Input: dimensioned drawing with shaded views. Units: mm. Origin: part minimum x, y, z. A direction names the side the tool comes from. Coordinates: 2 decimals unless noted, no trailing zeros. Order: outer loops, then holes, each group sorted by start corner. A loop starts at its lowest first (then second) coordinate and runs counter-clockwise, first axis right, second up. Notation, with made-up numbers: (-7, 73.25) - (36, 73.25) arc R33 cw to (36, 104.25) - close; hole circle Ø2 at (4, 58.25). An arc over 180 degrees is marked (long way). Answer as CSV lines item,"result". Start each with the question number.
Item 1: Draft query along X for the marked faces 4, 5 and 6. Return one class per face: +X half, -X half, draft (parallel to the pull), parting line (faces both ways), or undercut.
Item 2: Material intervals for line 1 along Z through (x, y) = (45, 38); line 2 along X through (y, z) = (35, 41.5); line 3 along Z through (x, y) = (40.5, 67), sorted ascending.
Item 3: First-contact query: pin 1 (5 mm diameter, centred on x = 32.5, z = 25, fed in from +Y); pin 2 (3 mm diameter, centred on x = 32.5, z = 17.5, fed in from +Y); pin 3 (1 mm diameter, centred on y = 44.5, z = 10.5, fed in from -X); pin 4 (4 mm diameter, centred on x = 36.5, y = 51, fed in from -Z). Flat tips, straight axial feed; report the tip coordinate or a pass-through.
Item 4: Access query for the marked faces 1, 2 and 3. Directions: +Z, -Z, +X, -X, +Y, -Y. A direction counts if a zero-diameter tool reaches every point of the face in a straight line with its end or side. Return the directions, or none.
Item 5: Section C-C (x = 38.1). Output: boundary loops of the cut face in (y, z).
Item 6: Section B-B (y = 47.5). Output: boundary loops of the cut face in (x, z).
Item 7: Section A-A (z = 36). Output: boundary loops of the cut face in (x, y).
Item 8: Section D-D (z = 8). Output: boundary loops of the cut face in (x, y), and give its area (3 significant figures).
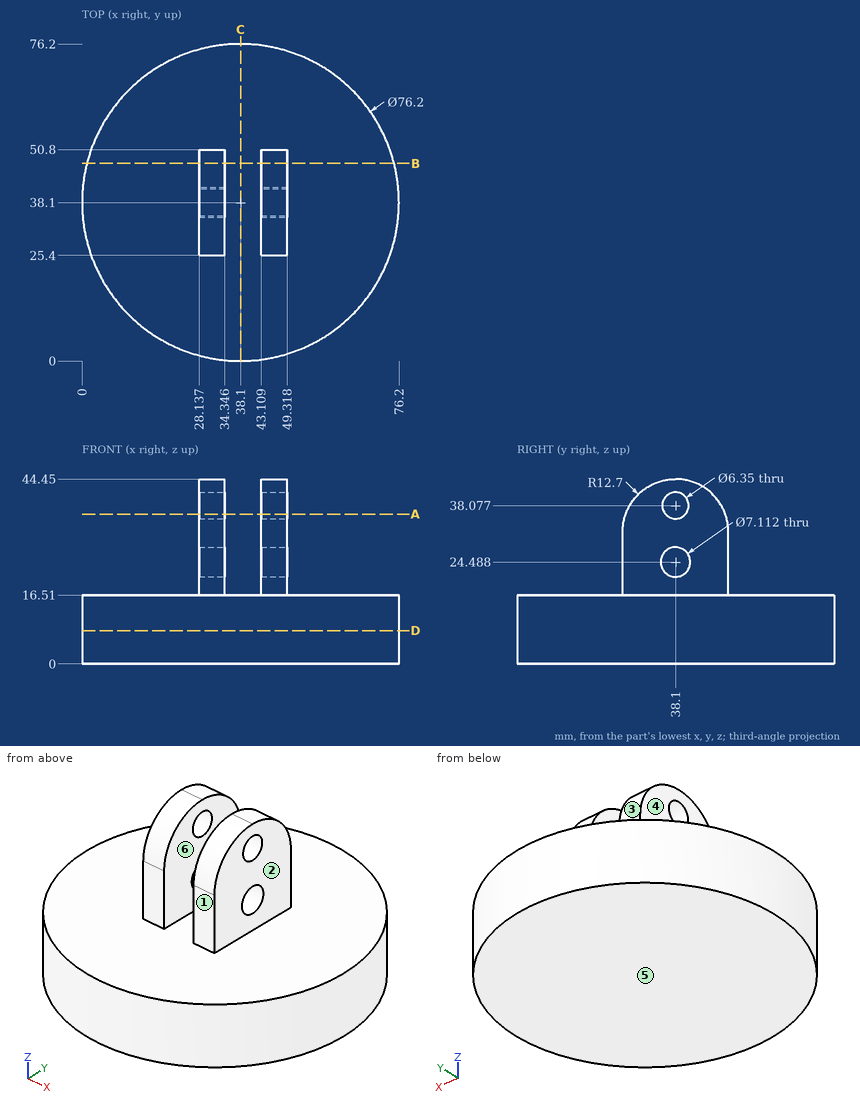
Determined:
1,face 4,"-X half"
1,face 5,"draft"
1,face 6,"undercut"
2,line 1,"z = 0 to 20.93, 28.04 to 34.9, 41.25 to 44.45"
2,line 2,"x = 28.14 to 34.35, 43.11 to 49.32"
2,line 3,"z = 0 to 16.51"
3,pin 1,"stops at y = 50.8"
3,pin 2,"stops at y = 75.94"
3,pin 3,"stops at x = 0.46"
3,pin 4,"stops at z = 0"
4,face 1,"+Z, +X, -X, -Y"
4,face 2,"+Z, +X, +Y, -Y"
4,face 3,"+Z, +X, -X, +Y"
5,outline,"(0, 0) - (76.2, 0) - (76.2, 16.51) - (0, 16.51) - close"
6,outline,"(1.18, 0) - (75.02, 0) - (75.02, 16.51) - (49.32, 16.51) - (49.32, 40.29) - (43.11, 40.29) - (43.11, 16.51) - (34.35, 16.51) - (34.35, 40.29) - (28.14, 40.29) - (28.14, 16.51) - (1.18, 16.51) - close"
7,outline,"(28.14, 26.13) - (34.35, 26.13) - (34.35, 35.7) - (28.14, 35.7) - close; (28.14, 40.5) - (34.35, 40.5) - (34.35, 50.07) - (28.14, 50.07) - close; (43.11, 26.13) - (49.32, 26.13) - (49.32, 35.7) - (43.11, 35.7) - close; (43.11, 40.5) - (49.32, 40.5) - (49.32, 50.07) - (43.11, 50.07) - close"
8,outline,"circle Ø76.2 at (38.1, 38.1)"
8,area,"4,560 mm^2"
